from build123d import *
from OCP.BRepFilletAPI import BRepFilletAPI_MakeFillet

# Parameters (mm, degrees)
SKETCH1_W                                           = 2.5
SKETCH1_H                                           = 6
BOSS_EXTRUDE1_DEPTH                                 = 6
SKETCH1_H_2                                         = 5.8
BOSS_EXTRUDE1_2_DEPTH                               = 6
BOSS_EXTRUDE1_3_DEPTH                               = 6
BOSS_EXTRUDE1_4_DEPTH                               = 6
SKETCH2_W                                           = 28
SKETCH2_H                                           = 45
BOSS_EXTRUDE2_DEPTH                                 = 2.5
BOSS_EXTRUDE3_DEPTH                                 = 2.5
CSK_FOR_M2_COUNTERSUNK_FLAT_HEAD_SCREW1_D           = 2.4
CSK_FOR_M2_COUNTERSUNK_FLAT_HEAD_SCREW1_DEPTH       = 4
CSK_FOR_M2_COUNTERSUNK_FLAT_HEAD_SCREW1_CSINK_D     = 4.4
CSK_FOR_M2_COUNTERSUNK_FLAT_HEAD_SCREW1_CSINK_ANGLE = 90
CSK_FOR_M2_COUNTERSUNK_FLAT_HEAD_SCREW1_TIP         = 0.721032743
CSK_FOR_M2_COUNTERSUNK_FLAT_HEAD_SCREW2_D           = 2.4
CSK_FOR_M2_COUNTERSUNK_FLAT_HEAD_SCREW2_DEPTH       = 4
CSK_FOR_M2_COUNTERSUNK_FLAT_HEAD_SCREW2_CSINK_D     = 4.4
CSK_FOR_M2_COUNTERSUNK_FLAT_HEAD_SCREW2_CSINK_ANGLE = 90
CSK_FOR_M2_COUNTERSUNK_FLAT_HEAD_SCREW2_TIP         = 0.721032743
FILLET1_R1                                          = 20
FILLET1_R2                                          = 5
FILLET2_R                                           = 1
FILLET3_R                                           = 0.5


with BuildPart() as part:
    # Sketch1 → Boss-Extrude1 (new body)
    with BuildSketch(Plane(origin=(30.100472417, 0, 0), x_dir=(0, 0, -1), z_dir=(1, 0, 0))):
        with Locations((-27.476835801, 55.903969126)):
            Rectangle(SKETCH1_W, SKETCH1_H)
    extrude(amount=BOSS_EXTRUDE1_DEPTH)



with BuildPart() as body_2:
    # Sketch1 → Boss-Extrude1 2 (new body)
    with BuildSketch(Plane(origin=(30.100472417, 0, 0), x_dir=(0, 0, -1), z_dir=(1, 0, 0))):
        with Locations((-27.476835801, 16.803969126)):
            Rectangle(SKETCH1_W, SKETCH1_H_2)
    extrude(amount=BOSS_EXTRUDE1_2_DEPTH)


with BuildPart() as body_3:
    # Sketch1 → Boss-Extrude1 3 (new body)
    with BuildSketch(Plane(origin=(30.100472417, 0, 0), x_dir=(0, 0, -1), z_dir=(1, 0, 0))):
        with Locations((-52.976835801, 16.803969126)):
            Rectangle(SKETCH1_W, SKETCH1_H_2)
    extrude(amount=BOSS_EXTRUDE1_3_DEPTH)


with BuildPart() as body_4:
    # Sketch1 → Boss-Extrude1 4 (new body)
    with BuildSketch(Plane(origin=(30.100472417, 0, 0), x_dir=(0, 0, -1), z_dir=(1, 0, 0))):
        with Locations((-52.976835801, 55.903969126)):
            Rectangle(SKETCH1_W, SKETCH1_H)
    extrude(amount=BOSS_EXTRUDE1_4_DEPTH)


with BuildPart() as part_1:
    add(part.part)

    add(body_2.part)  # Boss-Extrude2 merges body 2

    add(body_3.part)  # Boss-Extrude2 merges body 3

    add(body_4.part)  # Boss-Extrude2 merges body 4
    # Sketch2 → Boss-Extrude2 (add)
    with BuildSketch(Plane(origin=(36.100472417, 0, 0), x_dir=(0, 0, -1), z_dir=(1, 0, 0))):
        with Locations((-40.226835801, 36.403969126)):
            Rectangle(SKETCH2_W, SKETCH2_H)
    extrude(amount=BOSS_EXTRUDE2_DEPTH)

    # Sketch3 → Boss-Extrude3 (add)
    with BuildSketch(Plane(origin=(38.600472417, 0, 0), x_dir=(0, 0, -1), z_dir=(1, 0, 0))):
        Polygon((-68.326835801, 89.203969126), (-26.226835801, 89.203969126), (-26.226835801, 58.903969126), (-54.226835801, 58.903969126), (-54.226835801, 69.203969126), (-68.326835801, 69.203969126), align=None)
    extrude(amount=-BOSS_EXTRUDE3_DEPTH)

    # CSK for M2 Countersunk Flat Head Screw1
    with Locations(Plane.XY.offset(54.226835801)):
        with Locations((33.100472417, 55.903969126), (33.100472417, 16.903969126)):
            CounterSinkHole(CSK_FOR_M2_COUNTERSUNK_FLAT_HEAD_SCREW1_D / 2, CSK_FOR_M2_COUNTERSUNK_FLAT_HEAD_SCREW1_CSINK_D / 2, depth=CSK_FOR_M2_COUNTERSUNK_FLAT_HEAD_SCREW1_DEPTH, counter_sink_angle=CSK_FOR_M2_COUNTERSUNK_FLAT_HEAD_SCREW1_CSINK_ANGLE)
            with Locations((0, 0, -(CSK_FOR_M2_COUNTERSUNK_FLAT_HEAD_SCREW1_DEPTH + CSK_FOR_M2_COUNTERSUNK_FLAT_HEAD_SCREW1_TIP / 2))):  # 118° drill point
                Cone(0, CSK_FOR_M2_COUNTERSUNK_FLAT_HEAD_SCREW1_D / 2, CSK_FOR_M2_COUNTERSUNK_FLAT_HEAD_SCREW1_TIP, mode=Mode.SUBTRACT)

    # CSK for M2 Countersunk Flat Head Screw2
    with Locations(Plane(origin=(0, 0, 26.226835801), x_dir=(-1, 0, 0), z_dir=(0, 0, -1))):
        with Locations((-33.100472417, 55.903969126), (-33.100472417, 16.903969126)):
            CounterSinkHole(CSK_FOR_M2_COUNTERSUNK_FLAT_HEAD_SCREW2_D / 2, CSK_FOR_M2_COUNTERSUNK_FLAT_HEAD_SCREW2_CSINK_D / 2, depth=CSK_FOR_M2_COUNTERSUNK_FLAT_HEAD_SCREW2_DEPTH, counter_sink_angle=CSK_FOR_M2_COUNTERSUNK_FLAT_HEAD_SCREW2_CSINK_ANGLE)
            with Locations((0, 0, -(CSK_FOR_M2_COUNTERSUNK_FLAT_HEAD_SCREW2_DEPTH + CSK_FOR_M2_COUNTERSUNK_FLAT_HEAD_SCREW2_TIP / 2))):  # 118° drill point
                Cone(0, CSK_FOR_M2_COUNTERSUNK_FLAT_HEAD_SCREW2_D / 2, CSK_FOR_M2_COUNTERSUNK_FLAT_HEAD_SCREW2_TIP, mode=Mode.SUBTRACT)

    # Fillet1: one fillet with a radius per group of edges: ONE call of the kernel's fillet builder (fillet() takes one radius for all edges)
    fillet1_edges_1 = [part_1.edges().sort_by_distance(p)[0] for p in [
        (37.350472417, 89.203969126, 26.226835801),
    ]]
    fillet1_edges_2 = [part_1.edges().sort_by_distance(p)[0] for p in [
        (37.350472417, 69.203969126, 54.226835801),
    ]]
    fillet1 = BRepFilletAPI_MakeFillet(part_1.part.solid().wrapped)
    for e in fillet1_edges_1:
        fillet1.Add(FILLET1_R1, e.wrapped)
    for e in fillet1_edges_2:
        fillet1.Add(FILLET1_R2, e.wrapped)
    add(Compound.cast(fillet1.Shape()), mode=Mode.REPLACE)

    # Loft1: read off the stored shape, not the designer's step
    # Loft1: loft between two sections, ruled curve by curve
    loft1_from = [
        Edge.make_bspline([(36.19639036, 89.203969126, 88.326835801), (36.953966117, 87.719429888, 88.326835801), (37.561920044, 86.105994191, 88.326835801), (38.385620937, 82.729240829, 88.326835801), (38.600472417, 80.966962635, 88.326835801), (38.600472417, 77.440975617, 88.326835801), (38.385620937, 75.678697423, 88.326835801), (37.561920044, 72.30194406, 88.326835801), (36.953966117, 70.688508364, 88.326835801), (36.19639036, 69.203969126, 88.326835801)], [0, 0, 0, 0, 0.25, 0.25, 0.5, 0.5, 0.75, 0.75, 1, 1, 1, 1], 3),
        Edge.make_bspline([(33.920980493, 69.203969126, 88.326835801), (34.754313826, 70.647344799, 88.326835801), (35.433250093, 72.246533252, 88.326835801), (36.357078765, 75.632424009, 88.326835801), (36.600472417, 77.417641176, 88.326835801), (36.600472417, 80.990297075, 88.326835801), (36.357078765, 82.775514243, 88.326835801), (35.433250093, 86.161405, 88.326835801), (34.754313826, 87.760593453, 88.326835801), (33.920980493, 89.203969126, 88.326835801)], [0, 0, 0, 0, 0.25, 0.25, 0.5, 0.5, 0.75, 0.75, 1, 1, 1, 1], 3),
        Edge.make_line((33.920980493, 69.203969126, 88.326835801), (36.19639036, 69.203969126, 88.326835801)),
        Edge.make_line((33.920980493, 89.203969126, 88.326835801), (36.19639036, 89.203969126, 88.326835801)),
    ]
    loft1_to = [
        Edge.make_bspline([(38.600472417, 89.203969126, 68.326835801), (38.600472417, 87.537302459, 68.326835801), (38.600472417, 85.870635792, 68.326835801), (38.600472417, 82.537302459, 68.326835801), (38.600472417, 80.870635792, 68.326835801), (38.600472417, 77.537302459, 68.326835801), (38.600472417, 75.870635792, 68.326835801), (38.600472417, 72.537302459, 68.326835801), (38.600472417, 70.870635792, 68.326835801), (38.600472417, 69.203969126, 68.326835801)], [0, 0, 0, 0, 0.25, 0.25, 0.5, 0.5, 0.75, 0.75, 1, 1, 1, 1], 3),
        Edge.make_bspline([(36.100472417, 69.203969126, 68.326835801), (36.100472417, 70.870635792, 68.326835801), (36.100472417, 72.537302459, 68.326835801), (36.100472417, 75.870635792, 68.326835801), (36.100472417, 77.537302459, 68.326835801), (36.100472417, 80.870635792, 68.326835801), (36.100472417, 82.537302459, 68.326835801), (36.100472417, 85.870635792, 68.326835801), (36.100472417, 87.537302459, 68.326835801), (36.100472417, 89.203969126, 68.326835801)], [0, 0, 0, 0, 0.25, 0.25, 0.5, 0.5, 0.75, 0.75, 1, 1, 1, 1], 3),
        Edge.make_line((36.100472417, 69.203969126, 68.326835801), (38.600472417, 69.203969126, 68.326835801)),
        Edge.make_line((36.100472417, 89.203969126, 68.326835801), (38.600472417, 89.203969126, 68.326835801)),
    ]
    loft1 = Solid(Shell([*[Face.make_surface_from_curves(loft1_from[k], loft1_to[k]) for k in range(4)], Face(Wire(loft1_from)), Face(Wire(loft1_to))]))
    add(loft1)

    # Fillet2
    fillet2_edges = [part_1.edges().sort_by_distance(p)[0] for p in [
        (30.100472417, 58.903969126, 27.476835801),
        (30.100472417, 52.903969126, 27.476835801),
        (30.100472417, 19.703969126, 27.476835801),
        (30.100472417, 13.903969126, 27.476835801),
        (30.100472417, 13.903969126, 52.976835801),
        (30.100472417, 19.703969126, 52.976835801),
        (30.100472417, 52.903969126, 52.976835801),
        (30.100472417, 58.903969126, 52.976835801),
    ]]
    fillet(fillet2_edges, radius=FILLET2_R)

    # Fillet3
    # the kernel refuses this fillet: 0.5 mm, written as the material it takes off along each edge
    with BuildSketch(Plane(origin=(29.850472417, 52.903969126, 28.726835801), x_dir=(0, 1, 0), z_dir=(1, 0, 0)), Plane(origin=(29.850472417, 52.903969126, 51.726835801), x_dir=(0, 0, 1), z_dir=(1, 0, 0))) as fillet3_piece_1:
        with BuildLine():
            CenterArc((FILLET3_R, -FILLET3_R), FILLET3_R, 90, 90)
            Line((0, -FILLET3_R), (0, 0))
            Line((0, 0), (FILLET3_R, 0))
        make_face()
    extrude(amount=6.25, mode=Mode.SUBTRACT)
    with BuildSketch(Plane(origin=(39.850472417, 13.903969126, 26.226835801), x_dir=(0, 0, 1), z_dir=(-1, 0, 0)), Plane(origin=(39.850472417, 13.903969126, 54.226835801), x_dir=(0, 1, 0), z_dir=(-1, 0, 0))) as fillet3_piece_2:
        with BuildLine():
            CenterArc((FILLET3_R, FILLET3_R), FILLET3_R, 180, 90)
            Line((0, FILLET3_R), (0, 0))
            Line((0, 0), (FILLET3_R, 0))
        make_face()
    extrude(amount=10, mode=Mode.SUBTRACT)
    with BuildSketch(Plane(origin=(29.850472417, 19.703969126, 28.726835801), x_dir=(0, -1, 0), z_dir=(1, 0, 0)), Plane(origin=(29.850472417, 19.703969126, 51.726835801), x_dir=(0, 0, 1), z_dir=(1, 0, 0))) as fillet3_piece_3:
        with BuildLine():
            CenterArc((FILLET3_R, FILLET3_R), FILLET3_R, 180, 90)
            Line((0, FILLET3_R), (0, 0))
            Line((0, 0), (FILLET3_R, 0))
        make_face()
    extrude(amount=6.25, mode=Mode.SUBTRACT)


solid = part_1.part
Input: part model. Units: mm. Frame: model coordinates. A direction names the side the tool comes from. Coordinates: 2 decimals unless noted, no trailing zeros. Loops run counter-clockwise (first coordinate to the right, second up) from the corner with the lowest first, then second, coordinate; pieces in that order, holes last. Notation, with made-up numbers: (21, 68.25) - (74, 68.25) arc R24 cw to (74, 88.25) - close; hole circle Ø6 at (-26.75, 41). An arc over 180 degrees is marked (long way). Answer in a Markdown table with one row per item. Add a question column.
Item 1: Contact query for flat-ended pins moving along their axis: P1, Ø3, axis at x = 34.5, z = 27.5, coming from the +Y side; P2, Ø3, axis at x = 33.1, y = 16.9, coming from the +Z side; P3, Ø3.5, axis at x = 37, z = 79, coming from the -Y side. Output: stop coordinate, or through.
Item 2: Section query B-B on y = 21. Return the cut outline in (x, z), then the cut area to 3 significant figures.
Item 3: Access query for faces 5 (the cylindrical face through (32.46, 56.92, 52.47)), 6 (the flat face through (34, 52.904, 27)), 7 (the flat face through (33.1, 57.3, 28.727)), 8 (the flat face through (37, 69.204, 74)), 9 (the flat face through (34, 58.904, 27)). Directions: +Z, -Z, +X, -X, +Y, -Y. A direction counts if a zero-diameter tool reaches every point of the face in a straight line with its end or side. Return the directions, or none.
Item 4: Mould query, pull axis Z, two halves, no side actions, for faces 1 (the flat face through (32, 16, 51.727)), 2 (the flat face through (33.1, 57.3, 51.727)), 3 (the flat face through (34, 58.904, 53)), 4 (the cylindrical face through (37.33, 67.78, 55.73)). Classes: released by +Z, released by -Z, zero draft, split by the parting line, or undercut.
Item 5: Line query: line 1 along Z through (x, y) = (35.5, 19); line 2 along X through (y, z) = (74.5, 48.5); line 3 along Y through (x, z) = (37.25, 75.5). Output: solid intervals per line, ascending. Write a range as [from, to].
Item 6: Section query A-A on z = 48.5. Return the cut outline in (x, y), then the cut area to 3 significant figures.
Recorded:
| question | item | result |
|---|---|---|
| 1 | P1 | y = 58.9 |
| 1 | P2 | z = 53.53 |
| 1 | P3 | y = 69.2 |
| 2 | outline | (36.1, 26.23) - (38.6, 26.23) - (38.6, 54.23) - (36.1, 54.23) - close |
| 2 | area | 70.0 mm^2 |
| 3 | face 5 | +Z, -Z |
| 3 | face 6 | +Z, -Z, -X |
| 3 | face 7 | -X, +Y, -Y |
| 3 | face 8 | +Z, +X, -X, -Y |
| 3 | face 9 | +Z, -Z, -X, +Y |
| 4 | face 1 | undercut |
| 4 | face 2 | undercut |
| 4 | face 3 | zero draft |
| 4 | face 4 | released by +Z |
| 5 | line 1 | [26.23, 28.73], [51.73, 54.23] |
| 5 | line 2 | [36.1, 38.6] |
| 5 | line 3 | [69.2, 89.2] |
| 6 | outline | (36.1, 13.9) - (38.6, 13.9) - (38.6, 89.2) - (36.1, 89.2) - close |
| 6 | area | 188 mm^2 |
